```python
from build123d import *

# Parameters (mm, degrees)
F1_DEPTH = 0.75
F2_R     = 1.25
F3_DEPTH = 1.5
F4_W     = 11.25
F4_H     = 0.35
F4_H_2   = 6.9
F5_DEPTH = 3.4
F4_W_2   = 8
F4_H_3   = 4.5
F4_H_4   = 1.5
F6_DEPTH = 2.75
F4_W_3   = 1.4
F4_H_5   = 18
F4_W_4   = 3.3
F7_DEPTH = 1.5
F4_W_5   = 11.4
F4_H_6   = 12
F8_DEPTH = 1.5


with BuildPart() as f1:
    # F0 (on Right) → F1 (new body, symmetric)
    with BuildSketch(Plane.YZ):
        with BuildLine():
            Line((29.5, 15), (-29.5, 15))
            ThreePointArc((-29.5, 15), (-31.6213203436, 14.1213203436), (-32.5, 12))
            Line((-32.5, 12), (-32.5, -12))
            ThreePointArc((-32.5, -12), (-31.6213203436, -14.1213203436), (-29.5, -15))
            Line((-29.5, -15), (29.5, -15))
            ThreePointArc((29.5, -15), (31.6213203436, -14.1213203436), (32.5, -12))
            Line((32.5, -12), (32.5, 12))
            ThreePointArc((32.5, 12), (31.6213203436, 14.1213203436), (29.5, 15))
        make_face()
    extrude(amount=F1_DEPTH, both=True)

    # F2 (on face) → F3 (cut, through all)
    with BuildSketch(Plane.YZ.offset(0.75)):
        with Locations((-29, 11.5)):
            Circle(F2_R)
        with Locations((29, 11.5)):
            Circle(F2_R)
        with Locations((29, -11.5)):
            Circle(F2_R)
        with Locations((-29, -11.5)):
            Circle(F2_R)
    extrude(amount=-F3_DEPTH, mode=Mode.SUBTRACT)

    # F4 (on face) → F5 (join)
    with BuildSketch(Plane.YZ.offset(0.75)):
        with Locations((-20.1, -15.175)):
            Rectangle(F4_W, F4_H)
        with Locations((-20.1, -11.55)):
            Rectangle(F4_W, F4_H_2)
    extrude(amount=F5_DEPTH)

    # F4 (on face) → F6 (join)
    with BuildSketch(Plane.YZ.offset(0.75)):
        with Locations((8.9, -12.75)):
            Rectangle(F4_W_2, F4_H_3)
        with Locations((8.9, -15.75)):
            Rectangle(F4_W_2, F4_H_4)
        with Locations((21.5, -12.75)):
            Rectangle(F4_W_2, F4_H_3)
        with Locations((21.5, -15.75)):
            Rectangle(F4_W_2, F4_H_4)
    extrude(amount=F6_DEPTH)

    # F4 (on face) → F7 (join)
    with BuildSketch(Plane.YZ.offset(0.75)):
        with Locations((33.2, 0)):
            Rectangle(F4_W_3, F4_H_5)
        with Locations((30.85, 0)):
            Rectangle(F4_W_4, F4_H_5)
    extrude(amount=F7_DEPTH)

    # F4 (on face) → F8 (join)
    with BuildSketch(Plane.YZ.offset(0.75)):
        with Locations((-25, 1.9)):
            Rectangle(F4_W_5, F4_H_6)
    extrude(amount=F8_DEPTH)


solid = f1.part
```
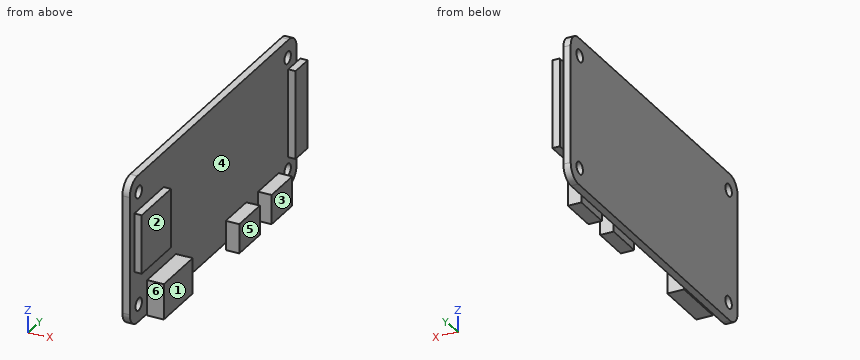
The listing builds one solid part. Answer for the finished solid, in the listing's coordinates (mm). Face numbers are marked on the shaded views. A direction names the side the tool comes from. Coordinates: 2 decimals unless noted, no trailing zeros. Loops run counter-clockwise (first coordinate to the right, second up) from the corner with the lowest first, then second, coordinate; pieces in that order, holes last. Notation, with made-up numbers: (87.25, 65) -> (106.25, 65) arc R17 cw to (106.25, 85) -> close; hole circle Ø8 at (27.5, 48). An arc over 180 degrees is marked (long way). Return JSON: item names as keys, results as strings. Group by question number.
(1) Determine the mould class of the marked faces 4, 5 and 6 for opening direction Y: released by +Y, released by -Y, zero draft, split by the parting line, or undercut.
(2) Which of the six approach directions +Z, -Z, +X, -X, +Y, -Y give full straight-line access (tool end or side, diameter ignored) to the marked faces 1, 2 and 3?
(3) A cutting plane is placed at B-B on z = -7.5. Write down the section's boundary in (x, y), and give its area (3 significant figures).
(4) A cutting plane is placed at C-C on z = 0.5. Write down the section's boundary in (x, y).
(5) A cutting plane is placed at D-D on y = -21. Write down the section's boundary in (x, z).
(6) Given pin 1 Ø2 at (x, z) = (2, -13) entering from +Y; pin 2 Ø1.5 at (y, z) = (-29, 11.5) entering from +X; pin 3 Ø2.5 at (y, z) = (31, 4) entering from +X; pin 4 Ø1.2 at (y, z) = (20.5, -16) entering from -X, each flat-ended and moving along its own axis, determine where each tip first touches the part or whether it passes through.
(7) A cutting plane is placed at A-A on y = 23. Write down the section's boundary in (x, z).
(8) Find the intervals of material crossed by probe 1 along Z at (x, y) = (-0.25, -29); probe 2 along Z at (x, y) = (0.9, -24); probe 3 along Y at (x, z) = (3, -11) (3 decimals), in increasing order. Write a range as from..to.
The answers:
{
 "1": {"face 4": "undercut", "face 5": "zero draft", "face 6": "released by -Y"},
 "2": {"face 1": "+Z, -Z, +X, +Y, -Y", "face 2": "+Z, +X, +Y, -Y", "face 3": "+Z, -Z, +X, +Y"},
 "3": {"outline": "(-0.75, -32.5) -> (0.75, -32.5) -> (0.75, 29.2) -> (2.25, 29.2) -> (2.25, 33.9) -> (0.75, 33.9) -> (0.75, 32.5) -> (-0.75, 32.5) -> close", "area": "105 mm^2"},
 "4": {"outline": "(-0.75, -32.5) -> (0.75, -32.5) -> (0.75, -30.7) -> (2.25, -30.7) -> (2.25, -19.3) -> (0.75, -19.3) -> (0.75, 29.2) -> (2.25, 29.2) -> (2.25, 33.9) -> (0.75, 33.9) -> (0.75, 32.5) -> (-0.75, 32.5) -> close"},
 "5": {"outline": "(-0.75, -15) -> (0.75, -15) -> (0.75, -15.35) -> (4.15, -15.35) -> (4.15, -8.1) -> (0.75, -8.1) -> (0.75, -4.1) -> (2.25, -4.1) -> (2.25, 7.9) -> (0.75, 7.9) -> (0.75, 15) -> (-0.75, 15) -> close"},
 "6": {"pin 1": "stops at y = 25.5", "pin 2": "passes through", "pin 3": "stops at x = 2.25", "pin 4": "stops at x = 0.75"},
 "7": {"outline": "(-0.75, -15) -> (0.75, -15) -> (0.75, -16.5) -> (3.5, -16.5) -> (3.5, -10.5) -> (0.75, -10.5) -> (0.75, 15) -> (-0.75, 15) -> close"},
 "8": {"probe 1": "z = -15..-12.75, -10.25..10.25, 12.75..15", "probe 2": "z = -15.35..-8.1, -4.1..7.9", "probe 3": "y = -25.725..-14.475, 4.9..12.9, 17.5..25.5"}
}
